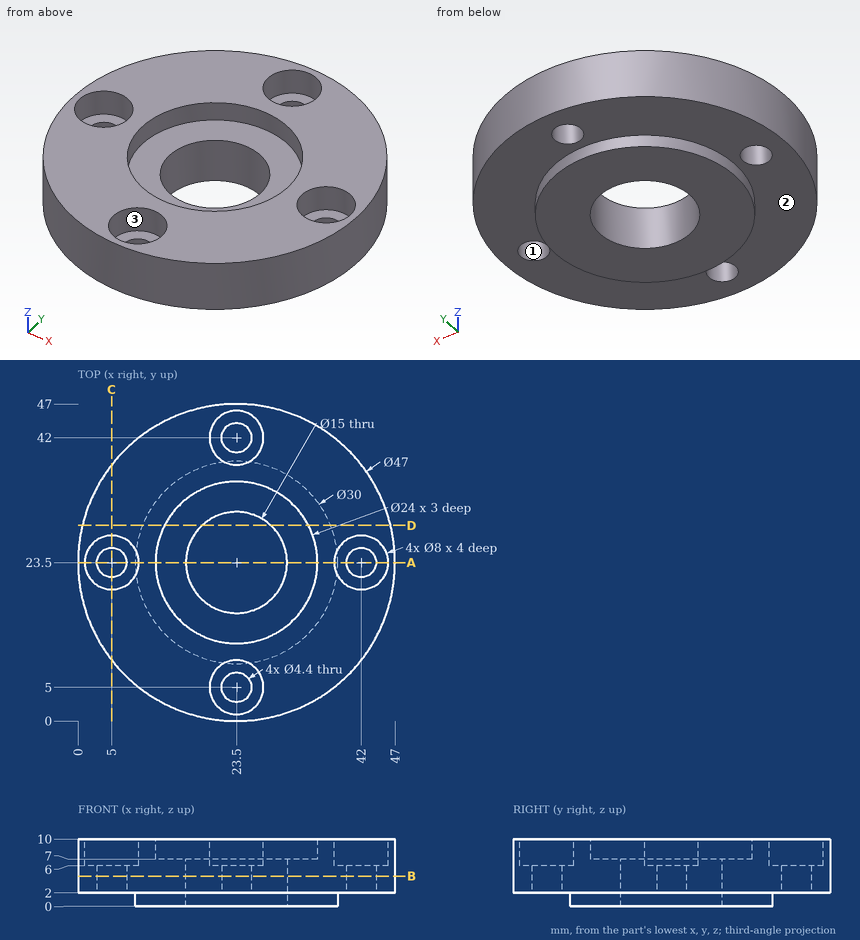
Check sheet for the drawn part. Datum: minimum x, y, z corner. Units: mm. A direction names the side the tool comes from. Coordinates: 2 decimals unless noted, no trailing zeros. Write each loop counter-clockwise with the first axis right and the second up, starting at its lowest first coordinate (ties: lowest second). Pieces come first, ordered by that corner, then holes. Notation, with made-up numbers: M 48.5,-39 L 75.5,-39 A16 ccw 75.5,-21 Z; hole C -24,-25 d6. An arc over 180 degrees is marked long. One line per item, written item: value.
Item 1: Section check A-A, the plane y = 23.5. State how many separate pieces and enclosed holes the cut face has, plus the area to 3 significant figures.
Check sheet entries:
separate pieces: 4
enclosed holes: 0
area: 160 mm^2
Item 2: Section check B-B, the plane z = 4.5. Record the boundary of the cut face in (x, y), plus the area to 3 significant figures.
Check sheet entries:
outline: C 23.5,23.5 d47; hole C 5,23.5 d4.4; hole C 23.5,23.5 d15; hole C 23.5,5 d4.4; hole C 23.5,42 d4.4; hole C 42,23.5 d4.4
area: 1,500 mm^2
Item 3: Gauge pin test, flat ends, axial feed: pin 1 Ø6 at (y, z) = (34, 5.5) entering from +X; pin 2 Ø2.5 at (x, y) = (43, 24.5) entering from +Z; pin 3 Ø5 at (x, z) = (20, 2) entering from -Y. Record the tip position at first contact, or that the pin passes through.
Check sheet entries:
pin 1: stops at x = 45.77
pin 2: stops at z = 6
pin 3: stops at y = 0.02
Item 4: Scan lines: line 1 along Y through (x, z) = (23.5, 3.5); line 2 along Y through (x, z) = (23.5, 7.5); line 3 along Y through (x, z) = (5, 4.4). Record each from-to range of solid material in increasing order.
Check sheet entries:
line 1: y = 0 to 2.8, 7.2 to 16, 31 to 39.8, 44.2 to 47
line 2: y = 0 to 1, 9 to 11.5, 35.5 to 38, 46 to 47
line 3: y = 9.01 to 21.3, 25.7 to 37.99
Item 5: Section check D-D, the plane y = 29. Record the boundary of the cut face in (x, z), plus the area to 3 significant figures.
Check sheet entries:
outline: M 0.65,2 L 9.54,2 L 9.54,0 L 18.4,0 L 18.4,7 L 12.83,7 L 12.83,10 L 0.65,10 Z; M 28.6,0 L 37.46,0 L 37.46,2 L 46.35,2 L 46.35,10 L 34.17,10 L 34.17,7 L 28.6,7 Z
area: 286 mm^2
Item 6: Section check C-C, the plane x = 5. Record the boundary of the cut face in (y, z), plus the area to 3 significant figures.
Check sheet entries:
outline: M 9.01,2 L 21.3,2 L 21.3,6 L 19.5,6 L 19.5,10 L 9.01,10 Z; M 25.7,2 L 37.99,2 L 37.99,10 L 27.5,10 L 27.5,6 L 25.7,6 Z
area: 182 mm^2
Item 7: Access from +Z, -Z, +X, -X, +Y, -Y to the whole of each face (thin tool, end or side, straight path). Record for the marked faces 1, 2 and 3.
Check sheet entries:
face 1: +Z, -Z
face 2: -Z
face 3: +Z
